CAD build for the part. Positions are in the model's coordinates, mm. A direction names the side the tool comes from. Coordinates: 2 decimals unless noted, no trailing zeros. Loops run counter-clockwise (first coordinate to the right, second up) from the corner with the lowest first, then second, coordinate; pieces in that order, holes last. Notation, with made-up numbers: (-9.75, 56) -> (37.25, 56) arc R33 cw to (37.25, 87) -> close; hole circle Ø9 at (61.25, 81.25). An arc over 180 degrees is marked (long way). Write each question's results on one line, items separated by ' | '.
```python
from build123d import *

# Parameters (mm, degrees)
F0_W     = 23
F0_H     = 38
F1_DEPTH = 175
F2_R     = 5
F4_DEPTH = 7
F5_W     = 4
F5_H     = 165
F6_DEPTH = 7


with BuildPart() as f1:
    # F0 (on Front) → F1 (new body)
    with BuildSketch(Plane.XZ):
        Rectangle(F0_W, F0_H)
    extrude(amount=F1_DEPTH)

    # F2
    f2_edges = [f1.edges().sort_by_distance(p)[0] for p in [
        (0, -175, 19),
        (0, -175, -19),
        (0, 0, 19),
        (0, 0, -19),
    ]]
    fillet(f2_edges, radius=F2_R)

    # F3 (on face) → F4 (cut)
    with BuildSketch(Plane(origin=(0, 0, -19), x_dir=(1, 0, 0), z_dir=(0, 0, -1))):
        Polygon((3.105181, 45.005862), (1.894584, 170), (-3.105181, 169.951576), (-1.894584, 44.957438), align=None)
    extrude(amount=-F4_DEPTH, mode=Mode.SUBTRACT)

    # F5 (on face) → F6 (cut)
    with BuildSketch(Plane.XY.offset(19)):
        with Locations((7.5, -87.5)):
            Rectangle(F5_W, F5_H)
    extrude(amount=-F6_DEPTH, mode=Mode.SUBTRACT)


solid = f1.part
```
Q1. Cut at A-A on y = -25. Write the cut outline in (x, z).
Results are:
outline: (-11.5, -19) -> (11.5, -19) -> (11.5, 19) -> (9.5, 19) -> (9.5, 12) -> (5.5, 12) -> (5.5, 19) -> (-11.5, 19) -> close
Q2. Wall check: L1, parallel to X at y = -144, z = 13; L2, parallel to Z at x = 8.25, y = -158; L3, parallel to Z at x = -0.75, y = -98. Give the ranges that are in metal, low to high. Write a range as from..to.
Results are:
L1: -11.5..5.5, 9.5..11.5 | L2: -19..12 | L3: -12..19
Q3. Pull direction X, two halves, no side cores. Call faces 1 (the flat face through (-11.5, -86, 0)), 2 (the flat face through (11.5, -86, 0)), 3 (the flat face through (7, -5, 16)), 4 (the flat face through (0, 0, 0)): +X half, -X half, draft (parallel to the pull), parting line (faces both ways), or undercut.
Results are:
face 1: -X half | face 2: +X half | face 3: undercut | face 4: draft
Q4. Drop flat-ended pins along their axis: pin 1 (1.9 mm diameter, centred on x = -1, y = -95.5, fed in from -Z); pin 2 (4.5 mm diameter, centred on x = 7.5, z = 17, fed in from +Y). Give the stop position or say it passes through.
Results are:
pin 1: z = -12 | pin 2: y = -0.06
Q5. Which spindle directions (+Z, -Z, +X, -X, +Y, -Y) get a long thin tool onto all of the face, cutting with end or side? Do faces 5 (the flat face through (0, -175, 0)), 6 (the flat face through (0, -108, -12)), 7 (the flat face through (7, -170, 16)). Say none if no direction does.
Results are:
face 5: +Z, -Z, +X, -X, -Y | face 6: -Z | face 7: +Z
Q6. Cut at C-C on y = -102.5. Write the cut outline in (x, z).
Results are:
outline: (-11.5, -19) -> (-2.45, -19) -> (-2.45, -12) -> (2.55, -12) -> (2.55, -19) -> (11.5, -19) -> (11.5, 19) -> (9.5, 19) -> (9.5, 12) -> (5.5, 12) -> (5.5, 19) -> (-11.5, 19) -> close
